```python
from build123d import *

# Parameters (mm, degrees)
SKETCH11_R          = 57.5
SKETCH11_R_2        = 44.5
BOSS_EXTRUDE3_DEPTH = 17
BOSS_EXTRUDE4_START = 1
SKETCH12_R          = 59
SKETCH12_R_2        = 44.5
BOSS_EXTRUDE4_DEPTH = 1
BOSS_EXTRUDE5_START = 17
SKETCH15_R          = 57.5
SKETCH15_R_2        = 44.5
BOSS_EXTRUDE5_DEPTH = 17


with BuildPart() as part:
    # Sketch10 → Revolve1 (revolve)
    with BuildSketch(Plane(origin=(0, 0, 0), x_dir=(1, 0, 0), z_dir=(0, 1, 0)), mode=Mode.PRIVATE) as revolve1_sk:
        Polygon((57.5, 17), (57.5, 0), (59, 0), align=None)
    revolve(revolve1_sk.sketch.rotate(Axis((0, 0, -66.869527167), (0, 0, 1)), 180), axis=Axis((0, 0, -66.869527167), (0, 0, 1)))

    # Sketch11 → Boss-Extrude3 (add)
    with BuildSketch(Plane.XY):
        Circle(SKETCH11_R)
        Circle(SKETCH11_R_2, mode=Mode.SUBTRACT)
    extrude(amount=-BOSS_EXTRUDE3_DEPTH)

    # Sketch12 → Boss-Extrude4 (add)
    with BuildSketch(Plane.XY.offset(BOSS_EXTRUDE4_START)):
        Circle(SKETCH12_R)
        Circle(SKETCH12_R_2, mode=Mode.SUBTRACT)
    boss_extrude4 = extrude(amount=-BOSS_EXTRUDE4_DEPTH)

    # Mirror11: Boss-Extrude4 across plane
    add(boss_extrude4.mirror(Plane.XY.offset(1)))

    # Sketch14 → Revolve2 (revolve)
    with BuildSketch(Plane(origin=(0, 0, 0), x_dir=(1, 0, 0), z_dir=(0, 1, 0)), mode=Mode.PRIVATE) as revolve2_sk:
        Polygon((-57.5, -2), (-57.5, -19), (-59, -1.968953878), align=None)
    revolve(revolve2_sk.sketch.rotate(Axis((0, 0, -34.208114596), (0, 0, 1)), 180), axis=Axis((0, 0, -34.208114596), (0, 0, 1)))

    # Sketch15 → Boss-Extrude5 (add)
    with BuildSketch(Plane.XY.offset(2).offset(BOSS_EXTRUDE5_START)):
        Circle(SKETCH15_R)
        Circle(SKETCH15_R_2, mode=Mode.SUBTRACT)
    extrude(amount=-BOSS_EXTRUDE5_DEPTH)


solid = part.part
```
Can you work these out from the model? Positions are in its coordinate system, mm. Give positions to 0.01 mm unless a question says otherwise; leave off trailing zeros. Loops run counter-clockwise (first coordinate to the right, second up) from the corner with the lowest first, then second, coordinate; pieces in that order, holes last. Notation, with made-up numbers: M -39.5,-7.75 L -9.5,-7.75 A25 ccw -9.5,26.25 Z; hole C 38.5,83 d6. An arc over 180 degrees is marked long. Use CSV: the item, a comma, the result in double quotes. Start each with the question number.
1. If I drill on L1, parallel to X at y = -32, z = -12.5; L2, parallel to Y at x = 2, z = 12.5; L3, parallel to Y at x = -28, z = -0.5, over which ranges is the centre line in solid material (lowest first)?
2. For P1, Ø1.5, axis at x = -17.5, z = 11.5, coming from the -Y side; P2, Ø1, axis at y = -35.5, z = 1, coming from the +X side; P3, Ø2, axis at x = -38, z = 3, coming from the +Y side, each with a flat end and sliding along its axis, tell me the tip position at first contact or that it passes through.
3. If we mould it in two halves opening along X, with no side actions, what happens to faces 1 (the face through (30, -34, 19)), 2 (the face through (-32.798, 30.075, 1.252)), 3 (the face through (-57.704, 2.54, 16.048))? For each: released by +X, released by -X, zero draft, split by the parting line, or undercut.
4. Imagine slicing it at C-C, the plane z = 13.5. Write out the boundary of the cut face in (x, y), plus the area to 3 significant figures.
5. Imagine slicing it at D-D, the plane z = -4.5. Write out the boundary of the cut face in (x, y).
Response values:
1,L1,"-48.25 to -30.92, 30.92 to 48.25"
1,L2,"-58.04 to -44.46, 44.46 to 58.04"
1,L3,"-51.88 to -34.59, 34.59 to 51.88"
2,P1,"y = -55.71"
2,P2,"x = 47.5"
2,P3,"y = 45.85"
3,face 1,"zero draft"
3,face 2,"undercut"
3,face 3,"split by the parting line"
4,outline,"C 0,0 d115.97; hole C 0,0 d89"
4,area,"4,340 mm^2"
5,outline,"C 0,0 d117.21; hole C 0,0 d89"
